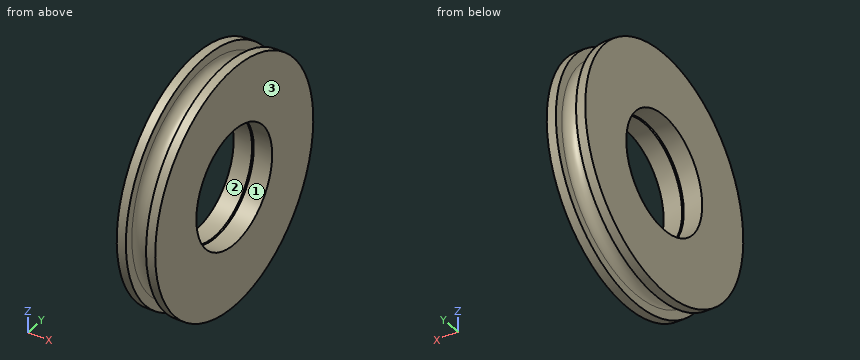
from build123d import *


with BuildPart() as part:
    # Sketch1 → Revolve1 (revolve)
    with BuildSketch(Plane(origin=(0, 0, 0), x_dir=(-1, 0, 0), z_dir=(0, 0, -1)), mode=Mode.PRIVATE) as revolve1_sk:
        with BuildLine():
            Line((4, 25), (2.1, 25))
            Line((2.1, 25), (2.1, 23.1))
            ThreePointArc((2.1, 23.1), (0, 21), (-2.1, 23.1))
            Line((-2.1, 23.1), (-2.1, 25))
            Line((-2.1, 25), (-4, 25))
            Line((-4, 25), (-4, 12))
            Line((-4, 12), (-0.173205081, 12))
            Line((-0.173205081, 12), (0, 12.3))
            Line((0, 12.3), (0.173205081, 12))
            Line((0.173205081, 12), (4, 12))
            Line((4, 12), (4, 25))
        make_face()
    revolve(revolve1_sk.sketch.rotate(Axis((3, 0, 0), (-1, 0, 0)), 270), axis=Axis((3, 0, 0), (-1, 0, 0)))


solid = part.part
CAD build for the part. Positions are in the model's coordinates, mm. Face numbers are marked on the shaded views. Round coordinates to 2 decimals unless told otherwise and drop trailing zeros. Order: outer loops, then holes, each group sorted by start corner. A loop starts at its lowest first (then second) coordinate and runs counter-clockwise, first axis right, second up. Notation, with made-up numbers: (29, -40) - (51, -40) arc R28 ccw to (51, -10) - close; hole circle Ø11 at (80.5, 49). An arc over 180 degrees is marked (long way). Return JSON: item names as keys, results as strings.
(1) Pull direction Z, two halves, no side cores. Call the marked faces 1, 2 and 3: +Z half, -Z half, draft (parallel to the pull), parting line (faces both ways), or undercut.
Answer key:
{"face 1": "undercut", "face 2": "undercut", "face 3": "draft"}
(2) Cut at C-C (x = 2.75). Give the cut face in (y, z), then the cut area to 3 significant figures.
Answer key:
{"outline": "circle Ø50 at (0, 0); hole circle Ø24 at (0, 0)", "area": "1,510 mm^2"}
(3) Pin check, flat tips, straight feed: pin 1 Ø15 at (y, z) = (1.5, -7) entering from +X; pin 2 Ø4 at (x, y) = (-0.5, -5.5) entering from -Z. Stop position of each tip, or through.
Answer key:
{"pin 1": "stops at x = 4", "pin 2": "stops at z = -24.63"}
(4) Wall check: probe 1 along Y at (x, z) = (3.5, 1.5); probe 2 along Y at (x, z) = (-3, -1); probe 3 along Z at (x, y) = (1.25, -1). Give the ranges that are in metal, low to high. Write a range as from..to.
Answer key:
{"probe 1": "y = -24.95..-11.91, 11.91..24.95", "probe 2": "y = -24.98..-11.96, 11.96..24.98", "probe 3": "z = -21.39..-11.96, 11.96..21.39"}
(5) Cut at A-A (z = 0). Give the cut face in (x, y), then the cut area to 3 significant figures.
Answer key:
{"outline": "(-4, -25) - (-2.1, -25) - (-2.1, -23.1) arc R2.1 cw to (2.1, -23.1) - (2.1, -25) - (4, -25) - (4, -12) - (0.17, -12) - (0, -12.3) - (-0.17, -12) - (-4, -12) - close; (-4, 12) - (-0.17, 12) - (0, 12.3) - (0.17, 12) - (4, 12) - (4, 25) - (2.1, 25) - (2.1, 23.1) arc R2.1 cw to (-2.1, 23.1) - (-2.1, 25) - (-4, 25) - close", "area": "178 mm^2"}
